Design review of the part built by this model. Coordinates are the model's own, in mm. Face numbers are marked on the shaded views. A direction names the side the tool comes from. Coordinates: 2 decimals unless noted, no trailing zeros. Answer in a Markdown table with one row per item.
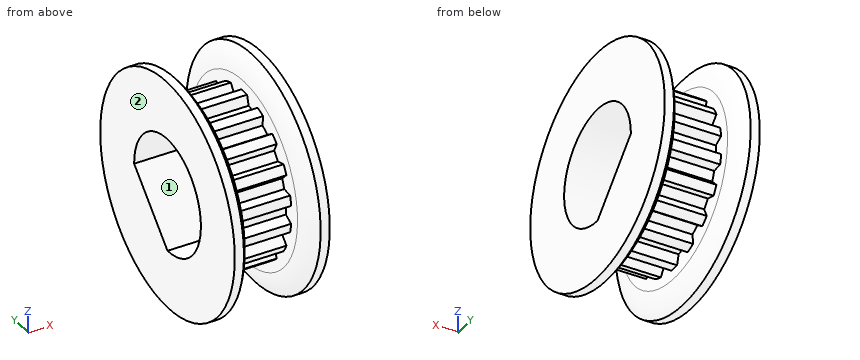
```python
from build123d import *

# Parameters (mm, degrees)
SKETCH4_R          = 5.8166
SKETCH4_R_2        = 5.65785
CUT_EXTRUDE2_DEPTH = 4.064
CUT_EXTRUDE1_DEPTH = 4.064
CIRPATTERN1_COUNT  = 18
SKETCH6_R          = 1.4605
CUT_EXTRUDE3_DEPTH = 13.95590486
CIRPATTERN2_COUNT  = 2
CIRPATTERN2_ANGLE  = 90
CUT_EXTRUDE5_REACH = 15.179
SKETCH9_R          = 8.0645
CUT_EXTRUDE6_REACH = 15.179
SKETCH10_R         = 2.38125


with BuildPart() as part:
    # Sketch1 → Revolve1 (revolve)
    with BuildSketch(Plane.XY, mode=Mode.PRIVATE) as revolve1_sk:
        with BuildLine():
            Line((-6.1468, 2.38125), (6.1468, 2.38125))
            Line((6.1468, 2.38125), (6.1468, 8.0645))
            Line((6.1468, 8.0645), (5.5118, 8.0645))
            ThreePointArc((5.5118, 8.0645), (5.040869168, 7.284417739), (4.8768, 6.3881))
            Line((4.8768, 6.3881), (4.8768, 5.8166))
            Line((4.8768, 5.8166), (0.8128, 5.8166))
            Line((0.8128, 5.8166), (0.8128, 6.3881))
            ThreePointArc((0.8128, 6.3881), (0.648730832, 7.284417739), (0.1778, 8.0645))
            Line((0.1778, 8.0645), (-0.4572, 8.0645))
            Line((-0.4572, 8.0645), (-0.4572, 3.9624))
            Line((-0.4572, 3.9624), (-6.1468, 3.9624))
            Line((-6.1468, 3.9624), (-6.1468, 2.38125))
        make_face()
    revolve(revolve1_sk.sketch.rotate(Axis((-6.1468, 0, 0), (1, 0, 0)), 90), axis=Axis((-6.1468, 0, 0), (1, 0, 0)))

    # Sketch4 → Cut-Extrude2 (cut)
    with BuildSketch(Plane(origin=(0.8128, 0, 0), x_dir=(0, 0, -1), z_dir=(1, 0, 0))):
        Circle(SKETCH4_R)
        Circle(SKETCH4_R_2, mode=Mode.SUBTRACT)
    extrude(amount=CUT_EXTRUDE2_DEPTH, mode=Mode.SUBTRACT)

    # Sketch3 → Cut-Extrude1 (cut)
    with BuildSketch(Plane(origin=(0.8128, 0, 0), x_dir=(0, 0, -1), z_dir=(1, 0, 0))):
        with BuildLine():
            Line((-0.64235315, 5.621267566), (-0.342998874, 4.97930025))
            Line((-0.342998874, 4.97930025), (0.342998874, 4.97930025))
            Line((0.342998874, 4.97930025), (0.64235315, 5.621267566))
            ThreePointArc((0.64235315, 5.621267566), (0, 5.65785), (-0.64235315, 5.621267566))
        make_face()
    cut_extrude1 = extrude(amount=CUT_EXTRUDE1_DEPTH, mode=Mode.SUBTRACT)

    # CirPattern1: Cut-Extrude1 ×18 about axis
    cirpattern1_axis = Axis((0, 0, 0), (1, 0, 0))
    for i in range(1, CIRPATTERN1_COUNT):
        add(cut_extrude1.rotate(cirpattern1_axis, i * 360 / CIRPATTERN1_COUNT), mode=Mode.SUBTRACT)

    # Sketch6 → Cut-Extrude3 (cut, through all)
    with BuildSketch(Plane(origin=(0, 0, 0), x_dir=(1, 0, 0), z_dir=(0, 1, 0))):
        with Locations(Location((-3.302, 0, 0), (0, 0, 90))):
            Circle(SKETCH6_R)
    cut_extrude3 = extrude(amount=CUT_EXTRUDE3_DEPTH, mode=Mode.SUBTRACT)

    # CirPattern2: Cut-Extrude3 ×2 about axis
    cirpattern2_axis = Axis((-6.1468, 0, 0), (1, 0, 0))
    for i in range(1, CIRPATTERN2_COUNT):
        add(cut_extrude3.rotate(cirpattern2_axis, i * CIRPATTERN2_ANGLE / (CIRPATTERN2_COUNT - 1)), mode=Mode.SUBTRACT)

    # Sketch9 → Cut-Extrude5 (cut, up to next)
    with BuildSketch(Plane.ZY.offset(0.4572), mode=Mode.PRIVATE) as cut_extrude5_sk1:
        Circle(SKETCH9_R)
    cut_extrude5_tool1 = extrude(cut_extrude5_sk1.sketch, amount=CUT_EXTRUDE5_REACH, mode=Mode.PRIVATE) & part.part
    add(cut_extrude5_tool1.solids().sort_by_distance((-0.4572, 0, 0))[0], mode=Mode.SUBTRACT)

    # Sketch10 → Cut-Extrude6 (cut, up to next)
    with BuildSketch(Plane(origin=(6.1468, 0, 0), x_dir=(0, 0, -1), z_dir=(1, 0, 0)), mode=Mode.PRIVATE) as cut_extrude6_sk1:
        with BuildLine():
            Line((4, 0), (0, 4))
            ThreePointArc((0, 4), (-2.828427125, -2.828427125), (4, 0))
        make_face()
        Circle(SKETCH10_R, mode=Mode.SUBTRACT)
    cut_extrude6_tool1 = extrude(cut_extrude6_sk1.sketch, amount=-CUT_EXTRUDE6_REACH, mode=Mode.PRIVATE) & part.part
    add(cut_extrude6_tool1.solids().sort_by_distance((6.1468, 1.92, -1.92))[0], mode=Mode.SUBTRACT)


solid = part.part
```
(1) For pin 1 (1.5 mm diameter, centred on y = -1, z = -1.5, fed in from -X); pin 2 (3 mm diameter, centred on x = 4.5, y = 5, fed in from +Z); pin 3 (1.5 mm diameter, centred on x = 3.5, z = 3.5, fed in from +Y); pin 4 (2 mm diameter, centred on x = 3, z = 3, fed in from -Y), all flat-tipped, find the tip position at first contact; note any pin that passes through.
Evaluation:
| item | result |
|---|---|
| pin 1 | passes through |
| pin 2 | stops at z = 7.06 |
| pin 3 | stops at y = 4.94 |
| pin 4 | stops at y = -5.06 |
(2) To check wall thickness, follow probe 1 along X at (y, z) = (0.75, 5.25); probe 2 along X at (y, z) = (6, 5); probe 3 along Y at (x, z) = (4, -2.75). State the ranges of each line that lie inside material, in increasing order.
Evaluation:
| item | result |
|---|---|
| probe 1 | x = -0.46 to 0.81, 4.88 to 6.15 |
| probe 2 | x = -0.46 to 0.38, 5.31 to 6.15 |
| probe 3 | y = -4.94 to -2.9, 1.25 to 4.94 |
(3) Tool access review of the marked faces 1 and 2: name each direction out of +Z, -Z, +X, -X, +Y, -Y from which nothing blocks a thin tool from reaching the whole face with its end or side.
Evaluation:
| item | result |
|---|---|
| face 1 | +X, -X |
| face 2 | +Z, -Z, -X, +Y, -Y |
